from build123d import *

# Parameters (mm, degrees)
SKETCH_R   = 2.25
SKETCH_R_2 = 3.25
PAD_DEPTH  = 6
FILLET_R   = 3


with BuildPart() as part:
    # Sketch → Pad (new body)
    with BuildSketch(Plane.XY):
        Polygon((0, 0), (25, 0), (25, 175), (12.374371, 187.374367), (0, 175), align=None)
        with Locations((12.5, 10)):
            Circle(SKETCH_R, mode=Mode.SUBTRACT)
        with Locations((12.5, 170)):
            Circle(SKETCH_R_2, mode=Mode.SUBTRACT)
    extrude(amount=PAD_DEPTH)

    # Fillet
    fillet_edges = [part.edges().sort_by_distance(p)[0] for p in [
        (12.374371, 187.374367, 3),
        (25, 175, 3),
        (0, 175, 3),
    ]]
    fillet(fillet_edges, radius=FILLET_R)


solid = part.part
Here's how the part is built. I have some questions about the finished solid (model axes, mm). Give positions to 0.01 mm unless a question says otherwise; leave off trailing zeros. Order: outer loops, then holes, each group sorted by start corner. A loop starts at its lowest first (then second) coordinate and runs counter-clockwise, first axis right, second up. Notation, with made-up numbers: M 27.5,11 L 35.5,11 A18 cw 35.5,21 Z; hole C -21.75,-4.5 d10. An arc over 180 degrees is marked long. Answer as a JSON object with one key per item and string values. Group by question number.
1) Suppose I cut it at C-C, the plane x = 12.5. Write out the boundary of the cut face in (y, z), plus the area to 3 significant figures.
2) Suppose I cut it at B-B, the plane y = 10. Write out the boundary of the cut face in (x, z).
3) I'm going to push a flat-ended pin straight in: pin 1 Ø4 at (x, y) = (12.5, 170) entering from +Z. Where does the tip first touch, or does it pass through?
4) Please list where these lines run through material, in increasing order: L1, parallel to Y at x = 12.5, z = 2.65; L2, parallel to X at y = 170, z = 2.6; L3, parallel to Y at x = 14.25, z = 1.95. Write a range as [from, to].
5) Suppose I cut it at A-A, the plane z = 2.6. Write out the boundary of the cut face in (x, y), plus the area to 3 significant figures.
6) We'd pull the mould along X, two halves only. Please class faces 1 (the flat face through (6, 181, 3)), 2 (the cylindrical face through (10.84, 11.52, 2.96)), 3 (the flat face through (19.365, 180.523, 2.958)): pulls with the +X half, pulls with the -X half, needs draft (parallel to the pull), parting line crosses it, or undercut.
7) Suppose I cut it at D-D, the plane y = 170. Write out the boundary of the cut face in (x, z).
Results found:
{
 "1": {"outline": "M 0,0 L 7.75,0 L 7.75,6 L 0,6 Z; M 12.25,0 L 166.75,0 L 166.75,6 L 12.25,6 Z; M 173.25,0 L 186.15,0 L 186.15,6 L 173.25,6 Z", "area": "1,050 mm²"},
 "2": {"outline": "M 0,0 L 10.25,0 L 10.25,6 L 0,6 Z; M 14.75,0 L 25,0 L 25,6 L 14.75,6 Z"},
 "3": {"pin 1": "through"},
 "4": {"L1": "[0, 7.75], [12.25, 166.75], [173.25, 186.15]", "L2": "[0, 9.25], [15.75, 25]", "L3": "[0, 8.59], [11.41, 167.26], [172.74, 185.51]"},
 "5": {"outline": "M 0,0 L 25,0 L 25,173.74 A3 ccw 24.1,175.88 L 14.5,185.3 A3 ccw 10.27,185.27 L 0.88,175.88 A3 ccw 0,173.76 Z; hole C 12.5,170 d6.5; hole C 12.5,10 d4.5", "area": "4,480 mm²"},
 "6": {"face 1": "pulls with the -X half", "face 2": "undercut", "face 3": "pulls with the +X half"},
 "7": {"outline": "M 0,0 L 9.25,0 L 9.25,6 L 0,6 Z; M 15.75,0 L 25,0 L 25,6 L 15.75,6 Z"}
}
